Check sheet for the modelled part. Datum: model origin and axes. Units: mm. A direction names the side the tool comes from. Coordinates: 2 decimals unless noted, no trailing zeros. Write each loop counter-clockwise with the first axis right and the second up, starting at its lowest first coordinate (ties: lowest second). Pieces come first, ordered by that corner, then holes. Notation, with made-up numbers: M 75,84 L 122,84 A28 cw 122,122 Z; hole C -35.5,57 d3. An arc over 180 degrees is marked long. Answer as CSV lines item,"result". Start each with the question number.
Q1. Sectioned sample at A-A, the plane y = 98. Record the cut outline in (x, z).
Q2. Access from +Z, -Z, +X, -X, +Y, -Y to the whole of each face (thin tool, end or side, straight path). Record for faces 5 (the flat face through (-153, 36.9, 4)), 6 (the cylindrical face through (-106.4, 153.6, 7)), 7 (the flat face through (-93, 33.01, 19)).
Q3. Sectioned sample at C-C, the plane y = 71. Record the cut outline in (x, z), then the cut area to 3 significant figures.
Q4. Sectioned sample at B-B, the plane x = -126.5. Record the cut outline in (y, z), then the cut area to 3 significant figures.
Q5. Sectioned sample at D-D, the plane z = 32. Count the separate pieces of the cut face and the enclosed holes in it, then the cut area to 3 significant figures.
Q6. Depth check by flat-ended pin: pin 1 Ø4 at (x, y) = (-46, 74) entering from -Z; pin 2 Ø9.5 at (y, z) = (135, 22.5) entering from -X; pin 3 Ø4 at (x, y) = (-32.44, 38.01) entering from +Z. Enter the tip coordinate at first touch or a pass-through.
Q7. Thickness scan on line 1 along Y through (x, z) = (-52.5, 15); line 2 along X through (y, z) = (57, 12); line 3 along X through (y, z) = (104, 35). Record the ranges inside material, lowest first. Write a range as from..to.
Q8. Mould release check, pull along Y, two halves, no side actions. Record for faces 1 (the cylindrical face through (-38.185, 43.872, 21.266)), 2 (the flat face through (-41, 105, 28)), 3 (the flat face through (-42.44, 36, 19)), 4 (the flat face through (-40.44, 153, 21)): pulls with the +Y half, pulls with the -Y half, needs draft (parallel to the pull), parting line crosses it, or undercut.
from build123d import *

# Parameters (mm, degrees)
ESQUISSE1_W                          = 126
ESQUISSE1_H                          = 126
BOSS_EXTRU_1_DEPTH                   = 40
ENL_V_MAT_EXTRU_1_DEPTH              = 38
ENL_V_MAT_EXTRU_2_REACH              = 223.428
ESQUISSE4_R                          = 1.75
ENL_V_MAT_EXTRU_5_DEPTH              = 36
COQUE1_DEPTH                         = 38
COQUE1_2_DEPTH                       = 2
BOSS_EXTRU_3_DEPTH                   = 2
ENL_V_MAT_EXTRU_6_REACH              = 228.297
ESQUISSE13_R                         = 1.75
ENL_V_MAT_EXTRU_14_DEPTH             = 2
ESQUISSE16_W                         = 40
ESQUISSE16_H                         = 72
ENL_V_MAT_EXTRU_9_DEPTH              = 2
BOSS_EXTRU_5_DEPTH                   = 2
ENL_V_MAT_EXTRU_11_REACH             = 228.968
ESQUISSE21_R                         = 2.5
ESQUISSE23_R                         = 3
BOSS_EXTRU_7_DEPTH                   = 10
ESQUISSE24_R                         = 1
ENL_V_MAT_EXTRU_12_DEPTH             = 9
R_P_TITION_LIN_AIRE1_COUNT           = 2
R_P_TITION_LIN_AIRE1_PITCH           = 25
R_P_TITION_LIN_AIRE2_COUNT           = 2
R_P_TITION_LIN_AIRE2_PITCH           = 52
R_P_TITION_LIN_AIRE2_COPY_1_SKETCH_R = 3
R_P_TITION_LIN_AIRE2_COPY_1_DEPTH    = 10
R_P_TITION_LIN_AIRE2_COPY_2_SKETCH_R = 1
R_P_TITION_LIN_AIRE2_COPY_2_DEPTH    = 9
ENL_V_MAT_EXTRU_13_REACH             = 211.939
ESQUISSE25_W                         = 10
ESQUISSE25_H                         = 15
ESQUISSE28_W                         = 2
ESQUISSE28_H                         = 72
BOSS_EXTRU_8_DEPTH                   = 3.5
ESQUISSE30_W                         = 20
ESQUISSE30_H                         = 5
BOSS_EXTRU_9_DEPTH                   = 38
ENL_V_MAT_EXTRU_15_REACH             = 218.201


# Read off the part's stored shape, not the designer's step: Coque1
with BuildPart() as part:
    # Esquisse1 → Boss.-Extru.1 (new body)
    with BuildSketch(Plane.XY):
        with Locations((-88.440384558, 94.010362694)):
            Rectangle(ESQUISSE1_W, ESQUISSE1_H)
    extrude(amount=BOSS_EXTRU_1_DEPTH)

    # Esquisse2 → Enlèv. mat.-Extru.1 (cut)
    with BuildSketch(Plane.XY.offset(40)):
        with BuildLine():
            Line((-40.440384558, 31.010362694), (-25.440384558, 31.010362694))
            Line((-25.440384558, 31.010362694), (-25.440384558, 46.010362694))
            Line((-25.440384558, 46.010362694), (-32.940384558, 46.010362694))
            ThreePointArc((-32.940384558, 46.010362694), (-38.243685417, 43.813663553), (-40.440384558, 38.510362694))
            Line((-40.440384558, 38.510362694), (-40.440384558, 31.010362694))
        make_face()
    enl_v_mat_extru_1 = extrude(amount=-ENL_V_MAT_EXTRU_1_DEPTH, mode=Mode.SUBTRACT)

    # Esquisse4 → Enlèv. mat.-Extru.2 (cut, up to next)
    with BuildSketch(Plane.XY.offset(2), mode=Mode.PRIVATE) as enl_v_mat_extru_2_sk1:
        with Locations((-32.440384558, 38.010362694)):
            Circle(ESQUISSE4_R)
    enl_v_mat_extru_2_tool1 = extrude(enl_v_mat_extru_2_sk1.sketch, amount=-ENL_V_MAT_EXTRU_2_REACH, mode=Mode.PRIVATE) & part.part
    enl_v_mat_extru_2 = enl_v_mat_extru_2_tool1.solids().sort_by_distance((-32.440385, 38.010363, 2))[0]
    add(enl_v_mat_extru_2, mode=Mode.SUBTRACT)

    # Symétrie1: Enlèv. mat.-Extru.1, Enlèv. mat.-Extru.2 across plane
    add(enl_v_mat_extru_1.mirror(Plane(origin=(0, 94.010362694, 0), x_dir=(0, 0, 1), z_dir=(0, -1, 0))), mode=Mode.SUBTRACT)
    add(enl_v_mat_extru_2.mirror(Plane(origin=(0, 94.010362694, 0), x_dir=(0, 0, 1), z_dir=(0, -1, 0))), mode=Mode.SUBTRACT)

    # Esquisse10 → Enlèv. mat.-Extru.5 (cut)
    with BuildSketch(Plane.XY.offset(40)):
        with BuildLine():
            Line((-151.440384558, 46.010362694), (-151.440384558, 31.010362694))
            Line((-151.440384558, 31.010362694), (-143.940384558, 31.010362694))
            Line((-143.940384558, 31.010362694), (-143.940384558, 38.510362694))
            ThreePointArc((-143.940384558, 38.510362694), (-146.137083699, 43.813663553), (-151.440384558, 46.010362694))
        make_face()
    enl_v_mat_extru_5 = extrude(amount=-ENL_V_MAT_EXTRU_5_DEPTH, mode=Mode.SUBTRACT)

    # Symétrie3: Enlèv. mat.-Extru.5 across plane
    add(enl_v_mat_extru_5.mirror(Plane(origin=(0, 94.010362694, 0), x_dir=(0, 0, 1), z_dir=(0, -1, 0))), mode=Mode.SUBTRACT)

    # Coque1 outline → Coque1 (cut)
    with BuildSketch(Plane.XY):
        with BuildLine():
            Line((-42.440384558, 155.010362694), (-141.940384558, 155.010362694))
            Line((-141.940384558, 155.010362694), (-141.940384558, 149.510362694))
            ThreePointArc((-141.940384558, 149.510362694), (-144.049511808, 143.541694501), (-149.440384558, 140.223274884))
            Line((-149.440384558, 140.223274884), (-149.440384558, 47.797450505))
            ThreePointArc((-149.440384558, 47.797450505), (-144.049511808, 44.479030887), (-141.940384558, 38.510362694))
            Line((-141.940384558, 38.510362694), (-141.940384558, 33.010362694))
            Line((-141.940384558, 33.010362694), (-42.440384558, 33.010362694))
            Line((-42.440384558, 33.010362694), (-42.440384558, 38.510362694))
            ThreePointArc((-42.440384558, 38.510362694), (-39.657898979, 45.227877116), (-32.940384558, 48.010362694))
            Line((-32.940384558, 48.010362694), (-27.440384558, 48.010362694))
            Line((-27.440384558, 48.010362694), (-27.440384558, 140.010362694))
            Line((-27.440384558, 140.010362694), (-32.940384558, 140.010362694))
            ThreePointArc((-32.940384558, 140.010362694), (-39.657898979, 142.792848273), (-42.440384558, 149.510362694))
            Line((-42.440384558, 149.510362694), (-42.440384558, 155.010362694))
        make_face()
    extrude(amount=COQUE1_DEPTH, mode=Mode.SUBTRACT)

    # Coque1 2 outline → Coque1 2 (cut)
    with BuildSketch(Plane.XY):
        with BuildLine():
            Line((-141.940384558, 155.010362694), (-149.440384558, 155.010362694))
            Line((-149.440384558, 155.010362694), (-149.440384558, 140.223274884))
            ThreePointArc((-149.440384558, 140.223274884), (-144.049511808, 143.541694501), (-141.940384558, 149.510362694))
            Line((-141.940384558, 149.510362694), (-141.940384558, 155.010362694))
        make_face()
        with BuildLine():
            ThreePointArc((-141.940384558, 38.510362694), (-144.049511808, 44.479030887), (-149.440384558, 47.797450505))
            Line((-149.440384558, 47.797450505), (-149.440384558, 33.010362694))
            Line((-149.440384558, 33.010362694), (-141.940384558, 33.010362694))
            Line((-141.940384558, 33.010362694), (-141.940384558, 38.510362694))
        make_face()
    extrude(amount=COQUE1_2_DEPTH, mode=Mode.SUBTRACT)

    # Esquisse12 → Boss.-Extru.3 (add)
    with BuildSketch(Plane.XY.offset(4)):
        with BuildLine():
            Line((-158.940384558, 31.010362694), (-158.940384558, 38.510362694))
            ThreePointArc((-158.940384558, 38.510362694), (-156.743685417, 43.813663553), (-151.440384558, 46.010362694))
            Line((-151.440384558, 46.010362694), (-151.440384558, 31.010362694))
            Line((-151.440384558, 31.010362694), (-158.940384558, 31.010362694))
        make_face()
    boss_extru_3 = extrude(amount=-BOSS_EXTRU_3_DEPTH)

    # Esquisse13 → Enlèv. mat.-Extru.6 (cut, up to next)
    with BuildSketch(Plane.XY.offset(4), mode=Mode.PRIVATE) as enl_v_mat_extru_6_sk1:
        with Locations((-151.440384558, 38.010362694)):
            Circle(ESQUISSE13_R)
    enl_v_mat_extru_6_tool1 = extrude(enl_v_mat_extru_6_sk1.sketch, amount=-ENL_V_MAT_EXTRU_6_REACH, mode=Mode.PRIVATE) & part.part
    enl_v_mat_extru_6 = enl_v_mat_extru_6_tool1.solids().sort_by_distance((-151.440385, 38.010363, 4))[0]
    add(enl_v_mat_extru_6, mode=Mode.SUBTRACT)

    # Esquisse27 → Enlèv. mat.-Extru.14 (cut)
    with BuildSketch(Plane(origin=(0, 0, 0), x_dir=(-1, 0, 0), z_dir=(0, 0, -1))):
        Polygon((149.440384558, 33.010362694), (149.440384558, 48.141426507), (151.440384558, 48.141426507), (151.440384558, 31.010362694), (142.02307923, 31.010362694), (142.041179779, 33.010362694), align=None)
    enl_v_mat_extru_14 = extrude(amount=-ENL_V_MAT_EXTRU_14_DEPTH, mode=Mode.SUBTRACT)

    # Symétrie5: Boss.-Extru.3, Enlèv. mat.-Extru.6, Enlèv. mat.-Extru.14 across plane
    add(boss_extru_3.mirror(Plane(origin=(0, 94.010362694, 0), x_dir=(0, 0, 1), z_dir=(0, -1, 0))))
    add(enl_v_mat_extru_6.mirror(Plane(origin=(0, 94.010362694, 0), x_dir=(0, 0, 1), z_dir=(0, -1, 0))), mode=Mode.SUBTRACT)
    add(enl_v_mat_extru_14.mirror(Plane(origin=(0, 94.010362694, 0), x_dir=(0, 0, 1), z_dir=(0, -1, 0))), mode=Mode.SUBTRACT)

    # Esquisse16 → Enlèv. mat.-Extru.9 (cut)
    with BuildSketch(Plane.ZY.offset(151.440384558)):
        with Locations((20, 94.010362694)):
            Rectangle(ESQUISSE16_W, ESQUISSE16_H)
    extrude(amount=-ENL_V_MAT_EXTRU_9_DEPTH, mode=Mode.SUBTRACT)

    # Esquisse20 → Boss.-Extru.5 (add)
    with BuildSketch(Plane.XY.offset(40)):
        with BuildLine():
            Line((-80.940384558, 31.010362694), (-95.940384558, 31.010362694))
            Line((-95.940384558, 31.010362694), (-95.940384558, 23.510362694))
            ThreePointArc((-95.940384558, 23.510362694), (-88.440384558, 16.010362694), (-80.940384558, 23.510362694))
            Line((-80.940384558, 23.510362694), (-80.940384558, 31.010362694))
        make_face()
    extrude(amount=-BOSS_EXTRU_5_DEPTH)

    # Esquisse21 → Enlèv. mat.-Extru.11 (cut, up to next)
    with BuildSketch(Plane.XY.offset(40), mode=Mode.PRIVATE) as enl_v_mat_extru_11_sk1:
        with Locations((-88.440384558, 23.760362694)):
            Circle(ESQUISSE21_R)
    enl_v_mat_extru_11_tool1 = extrude(enl_v_mat_extru_11_sk1.sketch, amount=-ENL_V_MAT_EXTRU_11_REACH, mode=Mode.PRIVATE) & part.part
    add(enl_v_mat_extru_11_tool1.solids().sort_by_distance((-88.440385, 23.760363, 40))[0], mode=Mode.SUBTRACT)

    # Esquisse23 → Boss.-Extru.7 (add)
    with BuildSketch(Plane(origin=(0, 0, 38), x_dir=(-1, 0, 0), z_dir=(0, 0, -1))):
        with Locations(Location((40.440384558, 81.010362694, 0), (0, 0, 180))):
            Circle(ESQUISSE23_R)
    boss_extru_7 = extrude(amount=BOSS_EXTRU_7_DEPTH)

    # Esquisse24 → Enlèv. mat.-Extru.12 (cut)
    with BuildSketch(Plane(origin=(0, 0, 28), x_dir=(-1, 0, 0), z_dir=(0, 0, -1))):
        with Locations((40.440384558, 81.010362694)):
            Circle(ESQUISSE24_R)
    enl_v_mat_extru_12 = extrude(amount=-ENL_V_MAT_EXTRU_12_DEPTH, mode=Mode.SUBTRACT)

    # Répétition linéaire1: Boss.-Extru.7, Enlèv. mat.-Extru.12 ×2
    with Locations(*[(0, i * R_P_TITION_LIN_AIRE1_PITCH, 0) for i in range(1, R_P_TITION_LIN_AIRE1_COUNT)]):
        add(boss_extru_7)
        add(enl_v_mat_extru_12, mode=Mode.SUBTRACT)

    # Répétition linéaire2: Boss.-Extru.7, Enlèv. mat.-Extru.12 ×2
    with Locations(*[(-i * R_P_TITION_LIN_AIRE2_PITCH, 0, 0) for i in range(1, R_P_TITION_LIN_AIRE2_COUNT)]):
        add(boss_extru_7)
        add(enl_v_mat_extru_12, mode=Mode.SUBTRACT)

    # Répétition linéaire2 copy 1 sketch → Répétition linéaire2 copy 1 (add)
    with BuildSketch(Plane(origin=(-52, 25, 38), x_dir=(-1, 0, 0), z_dir=(0, 0, -1))):
        with Locations(Location((40.440384558, 81.010362694, 0), (0, 0, 180))):
            Circle(R_P_TITION_LIN_AIRE2_COPY_1_SKETCH_R)
    extrude(amount=R_P_TITION_LIN_AIRE2_COPY_1_DEPTH)

    # Répétition linéaire2 copy 2 sketch → Répétition linéaire2 copy 2 (cut)
    with BuildSketch(Plane(origin=(-52, 25, 28), x_dir=(-1, 0, 0), z_dir=(0, 0, -1))):
        with Locations((40.440384558, 81.010362694)):
            Circle(R_P_TITION_LIN_AIRE2_COPY_2_SKETCH_R)
    extrude(amount=-R_P_TITION_LIN_AIRE2_COPY_2_DEPTH, mode=Mode.SUBTRACT)

    # Esquisse25 → Enlèv. mat.-Extru.13 (cut, up to next)
    with BuildSketch(Plane(origin=(-25.440384558, 0, 0), x_dir=(0, 0, -1), z_dir=(1, 0, 0)), mode=Mode.PRIVATE) as enl_v_mat_extru_13_sk1:
        with Locations((-13, 94.010362694)):
            Rectangle(ESQUISSE25_W, ESQUISSE25_H)
    enl_v_mat_extru_13_tool1 = extrude(enl_v_mat_extru_13_sk1.sketch, amount=-ENL_V_MAT_EXTRU_13_REACH, mode=Mode.PRIVATE) & part.part
    add(enl_v_mat_extru_13_tool1.solids().sort_by_distance((-25.440385, 94.010363, 13))[0], mode=Mode.SUBTRACT)

    # Esquisse28 → Boss.-Extru.8 (add)
    with BuildSketch(Plane.ZY.offset(149.440384558)):
        with Locations((39, 94.010362694)):
            Rectangle(ESQUISSE28_W, ESQUISSE28_H)
    extrude(amount=BOSS_EXTRU_8_DEPTH)

    # Esquisse30 → Boss.-Extru.9 (add)
    with BuildSketch(Plane(origin=(0, 0, 38), x_dir=(-1, 0, 0), z_dir=(0, 0, -1))):
        with Locations((106.440384558, 152.510362694)):
            Rectangle(ESQUISSE30_W, ESQUISSE30_H)
    extrude(amount=BOSS_EXTRU_9_DEPTH)

    # Esquisse29 → Enlèv. mat.-Extru.15 (cut, up to next)
    with BuildSketch(Plane(origin=(0, 157.010362694, 0), x_dir=(1, 0, 0), z_dir=(0, 1, 0)), mode=Mode.PRIVATE) as enl_v_mat_extru_15_sk1:
        with BuildLine():
            Line((-110.440384558, -3), (-110.440384558, 0))
            Line((-110.440384558, 0), (-102.440384558, 0))
            Line((-102.440384558, 0), (-102.440384558, -3))
            ThreePointArc((-102.440384558, -3), (-106.440384558, -7), (-110.440384558, -3))
        make_face()
    enl_v_mat_extru_15_tool1 = extrude(enl_v_mat_extru_15_sk1.sketch, amount=-ENL_V_MAT_EXTRU_15_REACH, mode=Mode.PRIVATE) & part.part
    add(enl_v_mat_extru_15_tool1.solids().sort_by_distance((-106.440385, 157.010363, 3.135687))[0], mode=Mode.SUBTRACT)


solid = part.part
Output:
1,outline,"M -152.94,38 L -27.44,38 L -27.44,18 L -25.44,18 L -25.44,40 L -152.94,40 Z; M -27.44,0 L -25.44,0 L -25.44,8 L -27.44,8 Z"
2,face 5,"+Z, -X, -Y"
2,face 6,"-Z, +Y"
2,face 7,"-Z"
3,outline,"M -152.94,38 L -27.44,38 L -27.44,0 L -25.44,0 L -25.44,40 L -152.94,40 Z"
3,area,"331 mm^2"
4,outline,"M 31.01,0 L 33.01,0 L 33.01,38 L 155.01,38 L 155.01,0 L 157.01,0 L 157.01,40 L 31.01,40 Z"
4,area,"404 mm^2"
5,separate pieces,"5"
5,enclosed holes,"4"
5,area,"1,020 mm^2"
6,pin 1,"stops at z = 38"
6,pin 2,"stops at x = -151.44"
6,pin 3,"stops at z = 2"
7,line 1,"y = 31.01..33.01, 155.01..157.01"
7,line 2,"x = -151.44..-149.44, -27.44..-25.44"
7,line 3,"x = -94.67..-90.21, -42.67..-38.21, -27.44..-25.44"
8,face 1,"pulls with the -Y half"
8,face 2,"undercut"
8,face 3,"undercut"
8,face 4,"needs draft"
